Drawing for the job (mm, zero at the part's lowest x, y, z). Coordinates: 2 decimals unless noted, no trailing zeros. Write each loop counter-clockwise with the first axis right and the second up, starting at its lowest first coordinate (ties: lowest second). Pieces come first, ordered by that corner, then holes. Notation, with made-up numbers: (-32.5, 57) -> (24.5, 57) arc R8 cw to (24.5, 70) -> close; hole circle Ø11 at (14.5, 29). An arc over 180 degrees is marked (long way). Write each question's results on one line, items separated by ' | '. Start each with the question number.
Q1. Two-plate mould, pull along X, no slides. Class the marked faces 1 and 2: released by +X, released by -X, zero draft, split by the parting line, or undercut.
Q2. Drill centre lines: line 1 (Y direction, x = 10, z = 1.65); line 2 (Y direction, x = 21.5, z = 1.5); line 3 (X direction, y = 24.5, z = 2.3). Where is each one in solid material? Low to high.
Q3. Saw through at B-B on z = 0.55. Count the separate pieces of the cut face and the enclosed holes in it, and give its area (3 significant figures).
Q4. Drop flat-ended pins along their axis: pin 1 Ø6 at (x, y) = (31, 20.5) entering from -Z; pin 2 Ø3 at (x, y) = (10, 26) entering from -Z. Give the stop position or say it passes through.
Q5. Saw through at A-A on y = 46. Give the cut face in (x, z), and give its area (3 significant figures).
Q6. Saw through at D-D on y = 30.5. Give the cut face in (x, z).
Q7. Saw through at C-C on x = 21.5. Give the cut face in (y, z), and give its area (3 significant figures).
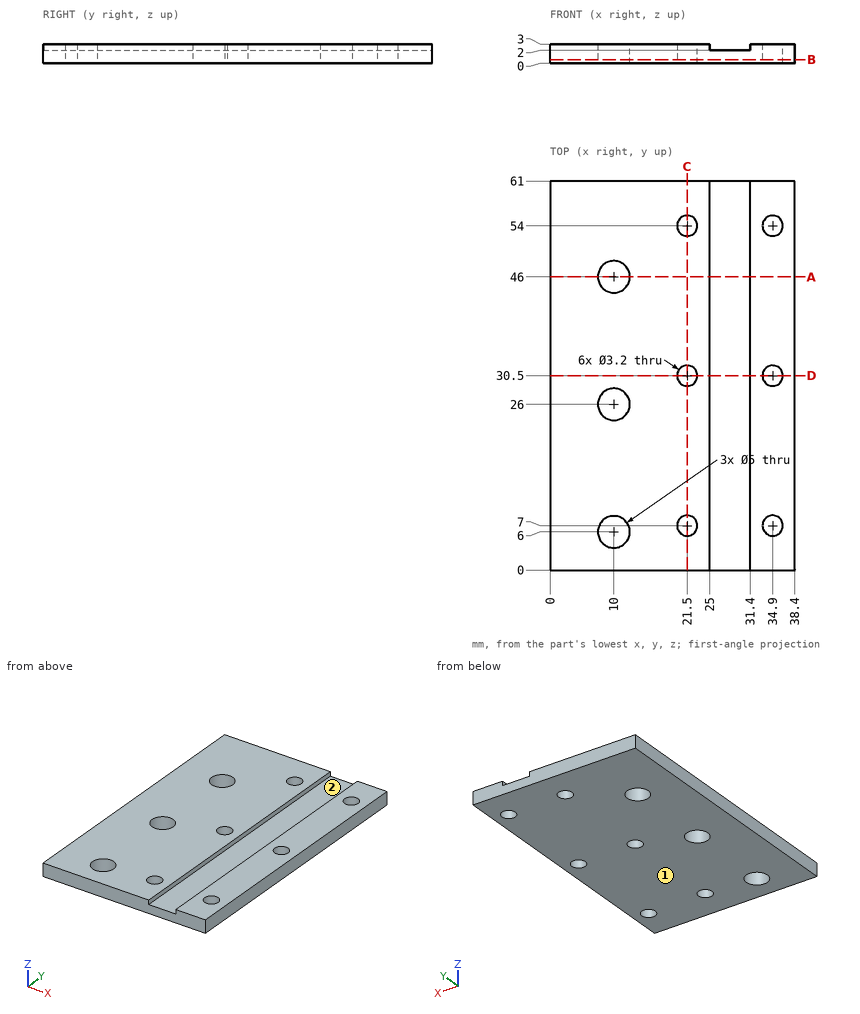
Returned:
1) face 1: zero draft | face 2: undercut
2) line 1: y = 0 to 3.5, 8.5 to 23.5, 28.5 to 43.5, 48.5 to 61 | line 2: y = 0 to 5.4, 8.6 to 28.9, 32.1 to 52.4, 55.6 to 61 | line 3: x = 0 to 8, 12 to 25, 31.4 to 38.4
3) separate pieces: 1 | enclosed holes: 9 | area: 2,240 mm2
4) pin 1: stops at z = 0 | pin 2: passes through
5) outline: (0, 0) -> (7.5, 0) -> (7.5, 3) -> (0, 3) -> close; (12.5, 0) -> (38.4, 0) -> (38.4, 3) -> (31.4, 3) -> (31.4, 2) -> (25, 2) -> (25, 3) -> (12.5, 3) -> close | area: 93.8 mm2
6) outline: (0, 0) -> (19.9, 0) -> (19.9, 3) -> (0, 3) -> close; (23.1, 0) -> (33.3, 0) -> (33.3, 3) -> (31.4, 3) -> (31.4, 2) -> (25, 2) -> (25, 3) -> (23.1, 3) -> close; (36.5, 0) -> (38.4, 0) -> (38.4, 3) -> (36.5, 3) -> close
7) outline: (0, 0) -> (5.4, 0) -> (5.4, 3) -> (0, 3) -> close; (8.6, 0) -> (28.9, 0) -> (28.9, 3) -> (8.6, 3) -> close; (32.1, 0) -> (52.4, 0) -> (52.4, 3) -> (32.1, 3) -> close; (55.6, 0) -> (61, 0) -> (61, 3) -> (55.6, 3) -> close | area: 154 mm2
